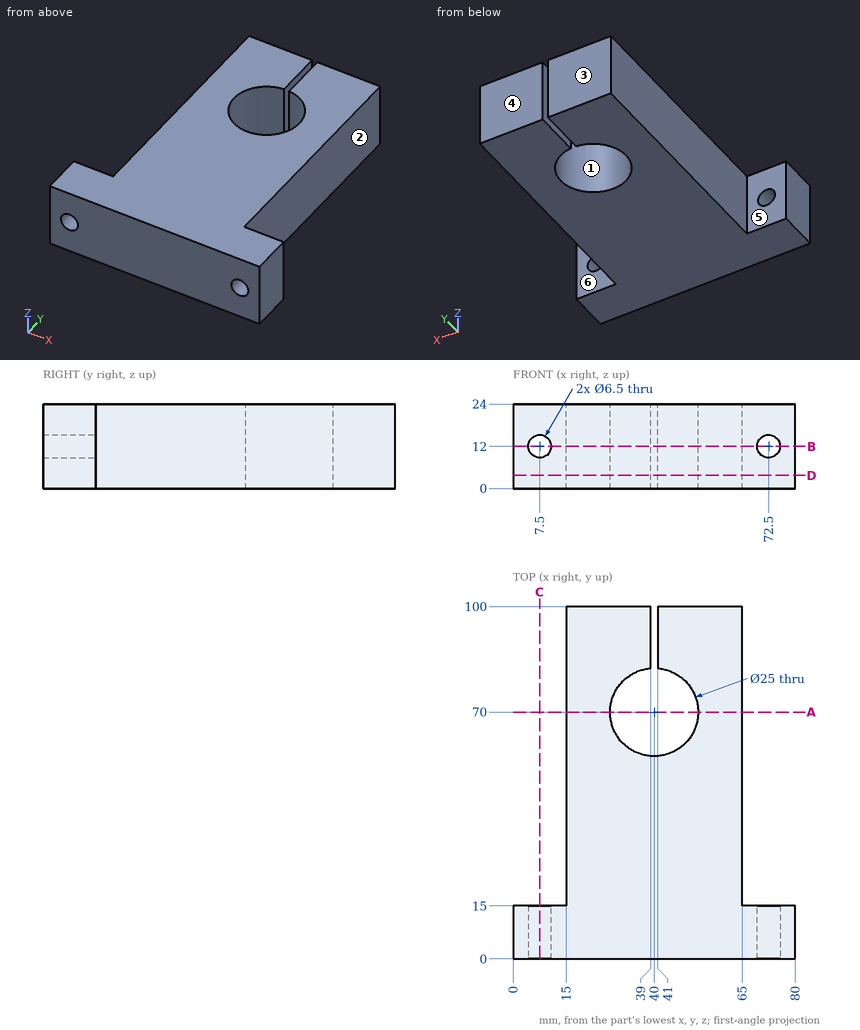
Can you work these out from the drawing? Everything is in mm from the part's minimum corner. A direction names the side the tool comes from. Give positions to 0.01 mm unless a question says otherwise; leave off trailing zeros. Loops run counter-clockwise (first coordinate to the right, second up) from the corner with the lowest first, then second, coordinate; pieces in that order, holes last. Notation, with made-up numbers: M 45,4 L 64,4 A21 ccw 64,21 Z; hole C 75.25,53 d2. An arc over 180 degrees is marked long. Put each result on its own line as item: value. Start each with the question number.
(1) If we mould it in two halves opening along X, with no side actions, what happens to the marked faces 1, 2 and 3? For each: +X half, -X half, draft (parallel to the pull), parting line (faces both ways), or undercut.
(2) I want a section at B-B on z = 12. Please give me the cut outline in (x, y), then the cut area to 3 significant figures.
(3) I want a section at C-C on x = 7.5. Please give me the cut outline in (y, z), then the cut area to 4 significant figures.
(4) I need wall thicknesses on line 1 along X through (y, z) = (70, 9); line 2 along Z through (x, y) = (72.5, 5); line 3 along X through (y, z) = (18.5, 6). Which ranges of each line are inside material? Lowest first, please. Write a range as [from, to].
(5) For the marked faces 4, 5 and 6, which set-ups out of +Z, -Z, +X, -X, +Y, -Y let a thin tool reach every point of the face, with its end or its side?
(6) I want a section at D-D on z = 3.75. Please give me the cut outline in (x, y).
(7) I want a section at A-A on y = 70. Please give me the cut outline in (x, z), then the cut area to 3 significant figures.
(8) Will these pins go through, and if not, where does the flat tip stop? pin 1 Ø5.5 at (y, z) = (88, 9.5) entering from +X; pin 2 Ø12 at (x, z) = (7, 13) entering from +Y; pin 3 Ø4 at (x, z) = (7.5, 12) entering from +Y; pin 4 Ø5.5 at (y, z) = (87.5, 7) entering from -X.
Answer block:
1. face 1: undercut
1. face 2: +X half
1. face 3: draft
2. outline: M 0,0 L 4.25,0 L 4.25,15 L 0,15 Z; M 10.75,0 L 69.25,0 L 69.25,15 L 65,15 L 65,100 L 41,100 L 41,82.46 A12.5 cw long 39,82.46 L 39,100 L 15,100 L 15,15 L 10.75,15 Z; M 75.75,0 L 80,0 L 80,15 L 75.75,15 Z
2. area: 4,730 mm^2
3. outline: M 0,0 L 15,0 L 15,8.75 L 0,8.75 Z; M 0,15.25 L 15,15.25 L 15,24 L 0,24 Z
3. area: 262.5 mm^2
4. line 1: [15, 27.5], [52.5, 65]
4. line 2: [0, 8.75], [15.25, 24]
4. line 3: [15, 65]
5. face 4: +Z, -Z, +X, -X, +Y
5. face 5: +Z, -Z, -X, +Y
5. face 6: +Z, -Z, +X, +Y
6. outline: M 0,0 L 80,0 L 80,15 L 65,15 L 65,100 L 41,100 L 41,82.46 A12.5 cw long 39,82.46 L 39,100 L 15,100 L 15,15 L 0,15 Z
7. outline: M 15,0 L 27.5,0 L 27.5,24 L 15,24 Z; M 52.5,0 L 65,0 L 65,24 L 52.5,24 Z
7. area: 600 mm^2
8. pin 1: x = 65
8. pin 2: y = 15
8. pin 3: through
8. pin 4: x = 15
